Verification items for the finished model (mm, model axes). Face numbers are marked on the shaded views. A direction names the side the tool comes from. Coordinates: 2 decimals unless noted, no trailing zeros. Write each loop counter-clockwise with the first axis right and the second up, starting at its lowest first coordinate (ties: lowest second). Pieces come first, ordered by that corner, then holes.
```python
from build123d import *

# Parameters (mm, degrees)
EXTRUDE_6_DEPTH     = 50
CUT_EXTRUDE_5_DEPTH = 63
EXTRUDE_7_DEPTH     = 15
FILLET_2_R          = 5
SKETCH_8_R          = 2.5
CUT_EXTRUDE_6_DEPTH = 10


with BuildPart() as part:
    # Эскиз2 → Бобышка-Вытянуть6 (new body)
    with BuildSketch(Plane.XY):
        Polygon((39.125, 45), (30, 45), (30, 0), (45, 0), align=None)
    extrude(amount=-EXTRUDE_6_DEPTH)

    # Эскиз4 → Вырез-Вытянуть5 (cut)
    with BuildSketch(Plane(origin=(0, 0, 0), x_dir=(0, 0, -1), z_dir=(1, 0, 0))):
        Polygon((50.288969981, 0), (35.288969981, 45), (50, 45), align=None)
        Polygon((0, 45), (0, 0), (30.288969981, 0), (15.293288519, 45), align=None)
    extrude(amount=CUT_EXTRUDE_5_DEPTH, mode=Mode.SUBTRACT)

    # Эскиз7 → Бобышка-Вытянуть7 (add)
    with BuildSketch(Plane.ZY.offset(-30)):
        Polygon((-50, 0), (-50, 0.866909943), (-48.622303314, 5), (-28.622783152, 5), (-30.288969981, 0), align=None)
    extrude(amount=EXTRUDE_7_DEPTH)

    # Скругление2
    fillet_2_edges = [part.edges().sort_by_distance(p)[0] for p in [
        (42.005910045, 22.933454971, -42.64448499),
    ]]
    fillet(fillet_2_edges, radius=FILLET_2_R)

    # Эскиз8 → Вырез-Вытянуть6 (cut)
    with BuildSketch(Plane(origin=(0, 5, 0), x_dir=(1, 0, 0), z_dir=(0, 1, 0))):
        with Locations((22.5, 38.622543233)):
            Circle(SKETCH_8_R)
    extrude(amount=-CUT_EXTRUDE_6_DEPTH, mode=Mode.SUBTRACT)


solid = part.part
```
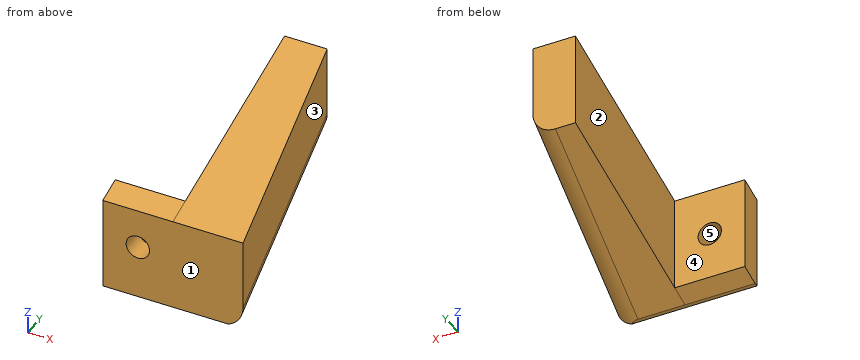
1. Sectioned sample at D-D, the plane x = 19. Record the boundary of the cut face in (y, z).
2. Draft check along X on the marked faces 3, 4 and 5. Enter one of: pulls with the +X half, pulls with the -X half, needs draft (parallel to the pull), parting line crosses it, or undercut.
3. Sectioned sample at A-A, the plane x = 22.5. Record the boundary of the cut face in (y, z), and give its area (3 significant figures).
4. Tool access check on the marked faces 1 and 2. Record the directions out of +Z, -Z, +X, -X, +Y, -Y that give a thin tool (end or side, any length) a straight path to the whole face; none if there is none.
5. Sectioned sample at B-B, the plane x = 31.75. Record the boundary of the cut face in (y, z).
6. Sectioned sample at C-C, the plane z = -24. Record the boundary of the cut face in (x, y) (3 decimals), and give its area (3 significant figures).
7. Gauge pin test, flat ends, axial feed: P1, Ø4.5, axis at x = 22.5, z = -38.62, coming from the -Y side; P2, Ø1.5, axis at y = 23, z = -37, coming from the +X side; P3, Ø12, axis at y = 25, z = -43, coming from the +X side; P4, Ø4, axis at x = 36.5, y = 8, coming from the +Z side. Record the tip position at first contact, or that the pin passes through.
8. Material ranges on L1, parallel to Z at x = 22.5, y = 2; L2, parallel to X at y = 43.5, z = -19.5; L3, parallel to X at y = 16.5, z = -42.5, recorded low to high.
Outcome:
1. outline: (0, -50) - (0.87, -50) - (5, -48.62) - (5, -28.62) - (0, -30.29) - close
2. face 3: pulls with the +X half
2. face 4: needs draft
2. face 5: undercut
3. outline: (0, -50) - (0.87, -50) - (5, -48.62) - (5, -41.12) - (0, -41.12) - close; (0, -36.12) - (5, -36.12) - (5, -28.62) - (0, -30.29) - close
3. area: 74.9 mm2
4. face 1: +Z, -Z, +X, -X, -Y
4. face 2: +Z, -Z, -X, +Y
5. outline: (0, -50) - (0.87, -50) - (45, -35.29) - (45, -15.29) - (0, -30.29) - close
6. outline: (30, 18.872) - (42.536, 18.872) - (39.125, 45) - (30, 45) - close
6. area: 283 mm2
7. P1: passes through
7. P2: stops at x = 42.1
7. P3: stops at x = 42.29
7. P4: stops at z = -26.96
8. L1: z = -49.62 to -41.12, -36.12 to -29.62
8. L2: x = 30 to 39.32
8. L3: x = 30 to 42.07
